Geometry: final body of the model. Coordinates: model frame, mm. A direction names the side the tool comes from. Round coordinates to 2 decimals unless told otherwise and drop trailing zeros. Write each loop counter-clockwise with the first axis right and the second up, starting at its lowest first coordinate (ties: lowest second). Pieces come first, ordered by that corner, then holes. Notation, with made-up numbers: M -37,2.5 L 2,2.5 A22 cw 2,12.5 Z; hole C 74,78.25 d7. An arc over 180 degrees is marked long. Put each result on its own line as item: value. Start each with the question number.
Autodesk Fusion 360 part; units mm, degrees
sketch "Sketch1" plane through (0, 0, 0) normal (0, 0, 1) x (1, 0, 0)
  circle A0 centre (0, 0) radius 7.5
  line L0 (-7.5, 0) -> (-7.5, -12.5)
  line L1 (-7.5, -12.5) -> (7.5, -12.5)
  line L2 (7.5, -12.5) -> (7.5, 0)
  circle A1 centre (0, 0) radius 4
  line L3 (-2, -12.5) -> (-2, -3.4641)
  line L4 (2, -3.4641) -> (2, -12.5)
  circle A2 centre (0, 0) radius 1.55
  circle A3 centre (0, 0) radius 2.75
  dimension "d1" = 15
  dimension "d2" = 20
  dimension "d3" = 8
  dimension "d4" = 4
  dimension "d5" = 3.1
  dimension "d6" = 5.5
extrude "Extrude1" add sketch "Sketch1" along normal blind 4 contours A0 A1 L3 L4 | A0 L1 L2 L4 | A0 L0 L1 L3 | A0 L1 L3 L4 | A0 A1 L3 L4 | A1 | A2 | A3
extrude "Extrude2" cut sketch "Sketch1" along normal blind 1.6 contours A0 L1 L3 L4 | A0 A1 L3 L4 | A1 | A2 | A3 picked at (0.436, -6.3069)
extrude "Extrude3" cut sketch "Sketch1" along normal through all contours A2
extrude "Extrude4" cut sketch "Sketch1" along normal up to surface (1.6 mm away) from surface at 2.4 contours A3
fillet "Fillet2" radius 5 2 edges at (2, -3.4641, 0.8) (-2, -3.4641, 0.8)
fillet "Fillet1" radius 0.8 5 edges at (2, -9.0784, 1.6) (2.286, -3.9902, 1.6) (0, 4, 1.6) (-2.286, -3.9902, 1.6) (-2, -9.0784, 1.6)
chamfer "Chamfer1" distance 2 angle 45 2 edges at (-7.5, -12.5, 2) (7.5, -12.5, 2)
chamfer "Chamfer2" distance 1 angle 45 6 edges at (-7.5, -5.25, 4) (7.5, -5.25, 4) (0, 7.5, 4) (0, -12.5, 4) (6.5, -11.5, 4) (-6.5, -11.5, 4)
cylinder "CylinderPrimitive1" add diameter 3.1 height -1.62 placed x (1, 0, 0) y (0, 1, 0) z (0, 0, 1) at (0, 0, 4)
equation "d12 = 4 mm - 1.6 mm"
1) First-contact query: pin 1 (2 mm diameter, centred on y = 5, z = 1.5, fed in from -X); pin 2 (2.5 mm diameter, centred on x = 0.5, y = 0, fed in from -Z). Flat tips, straight axial feed; report the tip coordinate or a pass-through.
2) Draft query along Y for faces 4 (the face through (-7, -11, 1)), 5 (the face through (1.77, -9.13, 1.36)), 6 (the face through (0.715, 1.375, 1.985)). Return one class per face: +Y half, -Y half, draft (parallel to the pull), parting line (faces both ways), or undercut.
3) Section C-C, the plane y = -8.5. Output: boundary loops of the cut face in (x, z), and give its area (3 significant figures).
4) Section B-B, the plane z = 3.65. Output: boundary loops of the cut face in (x, y).
5) Access query for faces 1 (the face through (0.715, -1.375, 3.211)), 2 (the face through (-1.77, -9.03, 1.36)), 3 (the face through (-2.28, -4.01, 0.41)). Directions: +Z, -Z, +X, -X, +Y, -Y. A direction counts if a zero-diameter tool reaches every point of the face in a straight line with its end or side. Return the directions, or none.
6) Ray query, probe 1 along Y at (x, z) = (0, 1.9); probe 2 along Y at (x, z) = (-0.5, 3.7); probe 3 along Y at (x, z) = (0, 3.3). Return the intervals inside material, ascending.
7) Section A-A, the plane x = 0. Output: boundary loops of the cut face in (y, z).
Solved:
1. pin 1: stops at x = -6.34
1. pin 2: stops at z = 1.6
2. face 4: -Y half
2. face 5: draft
2. face 6: undercut
3. outline: M -7.5,0 L -2,0 L -2,0.8 A0.8 cw -1.2,1.6 L 1.2,1.6 A0.8 cw 2,0.8 L 2,0 L 7.5,0 L 7.5,3 L 6.5,4 L -6.5,4 L -7.5,3 Z
3. area: 52.9 mm2
4. outline: M -6.85,-10.23 L -5.23,-11.85 L 5.23,-11.85 L 6.85,-10.23 L 6.85,0 A6.85 ccw -6.85,0 Z; C 0,0 d3.1; hole C 0,0 d5.5
5. face 1: +Z
5. face 2: -Z, -Y
5. face 3: -Z
6. probe 1: y = -12.5 to -1.55, 1.55 to 7.5
6. probe 2: y = -11.8 to -2.7, -1.47 to 1.47, 2.7 to 6.78
6. probe 3: y = -12.2 to -2.75, -1.55 to 1.55, 2.75 to 7.2
7. outline: M -12.5,1.6 L -1.55,1.6 L -1.55,2.38 L 1.55,2.38 L 1.55,1.6 L 3.2,1.6 A0.8 cw 4,0.8 L 4,0 L 7.5,0 L 7.5,3 L 6.5,4 L 2.75,4 L 2.75,2.4 L 1.55,2.4 L 1.55,4 L -1.55,4 L -1.55,2.4 L -2.75,2.4 L -2.75,4 L -11.5,4 L -12.5,3 Z
